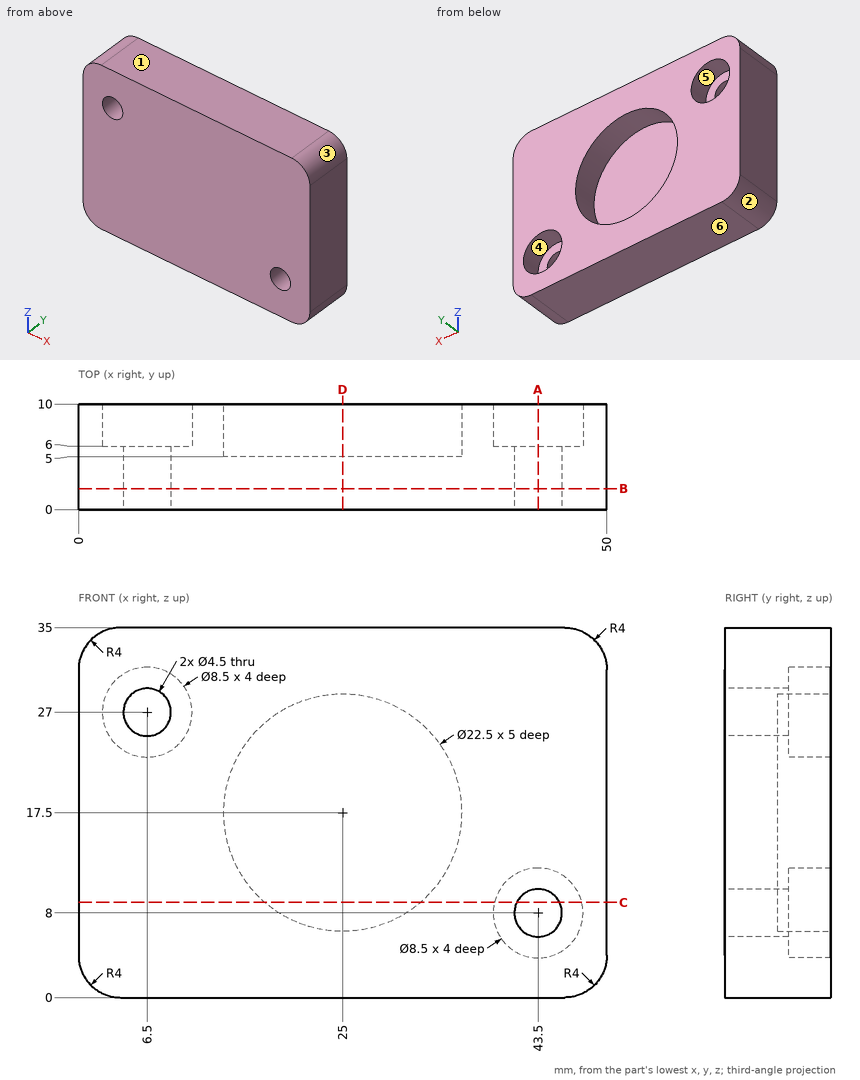
Answer from the drawing. Dimensions are ordinates in mm from the lowest x, y and z of the part. A direction names the side the tool comes from. Round coordinates to 2 decimals unless told otherwise and drop trailing zeros. Order: outer loops, then holes, each group sorted by start corner. A loop starts at its lowest first (then second) coordinate and runs counter-clockwise, first axis right, second up.
1) For the marked faces 5 and 6, determine the directions among +Z, -Z, +X, -X, +Y, -Y from which every point of the face is accessible in a straight line to the end or side of a thin tool.
2) The part is cut by section C-C on z = 9. Write down the section's boundary in (x, y), plus the area to 3 significant figures.
3) The part is cut by section B-B on y = 2. Write down the section's boundary in (x, z).
4) Flat-ended cylindrical pins translate along their axes: pin 1 (4 mm diameter, centred on x = 41.5, z = 8, fed in from +Y); pin 2 (4 mm diameter, centred on x = 6.5, z = 27, fed in from +Y). Find the tip coordinate at first contact, or state that the pin passes through.
5) The mould has two halves that part along X. Classify the marked faces 1, 2, 3 and 4: released by +X, released by -X, zero draft, split by the parting line, or undercut.
6) The part is cut by section D-D on x = 25. Write down the section's boundary in (y, z).
7) Straight lines are drawn through the part: L1, parallel to X at y = 6.9, z = 17.5; L2, parallel to Z at x = 6.5, y = 4.5; L3, parallel to X at y = 6.5, z = 8. For each, find the intervals that lie inside material, in ascending order.
8) The part is cut by section A-A on x = 43.5. Write down the section's boundary in (y, z).
Resolved:
1. face 5: +Y
1. face 6: -Z, +X, -X, +Y, -Y
2. outline: (0, 0) - (41.48, 0) - (41.48, 6) - (39.37, 6) - (39.37, 10) - (32.37, 10) - (32.37, 5) - (17.63, 5) - (17.63, 10) - (0, 10) - close; (45.52, 0) - (50, 0) - (50, 10) - (47.63, 10) - (47.63, 6) - (45.52, 6) - close
2. area: 369 mm2
3. outline: (0, 4) arc R4 ccw to (4, 0) - (46, 0) arc R4 ccw to (50, 4) - (50, 31) arc R4 ccw to (46, 35) - (4, 35) arc R4 ccw to (0, 31) - close; hole circle Ø4.5 at (6.5, 27); hole circle Ø4.5 at (43.5, 8)
4. pin 1: stops at y = 6
4. pin 2: passes through
5. face 1: zero draft
5. face 2: released by -X
5. face 3: released by +X
5. face 4: undercut
6. outline: (0, 0) - (10, 0) - (10, 6.25) - (5, 6.25) - (5, 28.75) - (10, 28.75) - (10, 35) - (0, 35) - close
7. L1: x = 0 to 13.75, 36.25 to 50
7. L2: z = 0 to 24.75, 29.25 to 35
7. L3: x = 0 to 18.97, 31.03 to 39.25, 47.75 to 50
8. outline: (0, 0) - (10, 0) - (10, 3.75) - (6, 3.75) - (6, 5.75) - (0, 5.75) - close; (0, 10.25) - (6, 10.25) - (6, 12.25) - (10, 12.25) - (10, 35) - (0, 35) - close
